Geometry: final body of the model. Coordinates: model frame, mm. Coordinates: 2 decimals unless noted, no trailing zeros. Order: outer loops, then holes, each group sorted by start corner. A loop starts at its lowest first (then second) coordinate and runs counter-clockwise, first axis right, second up. Notation, with made-up numbers: M 11.5,-8.5 L 39.5,-8.5 A14 cw 39.5,5.5 Z; hole C 33,-2.5 d7. An arc over 180 degrees is marked long. One line per question, with ' | ' between items.
from build123d import *

# Parameters (mm, degrees)
F0_W     = 100
F0_H     = 40
F0_R     = 7.5
F1_DEPTH = 25
F2_R     = 2.5
F2_R_2   = 2.193335
F3_DEPTH = 40.001
F4_R     = 5


with BuildPart() as f1:
    # F0 (on Front) → F1 (new body)
    with BuildSketch(Plane.XZ):
        Rectangle(F0_W, F0_H)
        with Locations((-27.932694, 0)):
            Circle(F0_R, mode=Mode.SUBTRACT)
        with Locations((23.894234, 0)):
            Circle(F0_R, mode=Mode.SUBTRACT)
    extrude(amount=F1_DEPTH)

    # F2 (on face) → F3 (cut, through all)
    with BuildSketch(Plane.XY.offset(20)):
        with Locations((-45, -12.810267)):
            Circle(F2_R)
        with Locations((45, -13.836424)):
            Circle(F2_R_2)
    extrude(amount=-F3_DEPTH, mode=Mode.SUBTRACT)

    # F4
    f4_edges = [f1.edges().sort_by_distance(p)[0] for p in [
        (-50, -25, 0),
        (0, -25, 20),
        (50, -25, 0),
    ]]
    fillet(f4_edges, radius=F4_R)


solid = f1.part
1. Section D-D, the plane x = 20. Output: boundary loops of the cut face in (y, z).
Response values:
outline: M -25,-20 L 0,-20 L 0,-6.41 L -25,-6.41 Z; M -25,6.41 L 0,6.41 L 0,20 L -20,20 A5 ccw -25,15 Z
2. Section B-B, the plane x = 30. Output: boundary loops of the cut face in (y, z).
Response values:
outline: M -25,-20 L 0,-20 L 0,-4.36 L -25,-4.36 Z; M -25,4.36 L 0,4.36 L 0,20 L -20,20 A5 ccw -25,15 Z
3. Section C-C, the plane y = -7.75. Output: boundary loops of the cut face in (x, z).
Response values:
outline: M -50,-20 L 50,-20 L 50,20 L -50,20 Z; hole C -27.93,0 d15; hole C 23.89,0 d15
4. Section A-A, the plane z = 0. Output: boundary loops of the cut face in (x, y).
Response values:
outline: M -50,-20 A5 ccw -45,-25 L -35.43,-25 L -35.43,0 L -50,0 Z; M -20.43,-25 L 16.39,-25 L 16.39,0 L -20.43,0 Z; M 31.39,-25 L 45,-25 A5 ccw 50,-20 L 50,0 L 31.39,0 Z; hole C -45,-12.81 d5; hole C 45,-13.84 d4.39
5. Material intervals for line 1 (X direction, y = -6.5, z = -0.5); line 2 (Y direction, x = -45, z = -9); line 3 (X direction, y = -13, z = -2), sorted ascending. Write a range as [from, to].
Response values:
line 1: x = [-50, -35.42], [-20.45, 16.41], [31.38, 50] | line 2: y = [-25, -15.31], [-10.31, 0] | line 3: x = [-50, -47.49], [-42.51, -35.16], [-20.7, 16.67], [31.12, 42.97], [47.03, 50]
6. Draft query along Z for faces 1 (the face through (-35.425, -12.325, 0.33)), 2 (the face through (-1, -12, -20)), 3 (the face through (-1, -10, 20)). Return one class per face: pulls with the +Z half, pulls with the -Z half, needs draft (parallel to the pull), parting line crosses it, or undercut.
Response values:
face 1: undercut | face 2: pulls with the -Z half | face 3: pulls with the +Z half
